```python
from build123d import *

# Parameters (mm, degrees)
SKETCH_1_W          = 49.5
SKETCH_1_H          = 24.5
EXTRUDE_1_DEPTH     = 22.5
SKETCH_2_R          = 2.5
CUT_EXTRUDE_1_DEPTH = 3
SKETCH_3_W          = 15.2
SKETCH_3_H          = 2.5
CUT_EXTRUDE_2_DEPTH = 8
CUT_EXTRUDE_3_DEPTH = 50
CUT_EXTRUDE_START   = 22.5
SKETCH_5_R          = 1.45
CUT_EXTRUDE_4_DEPTH = 10
FILLET_1_R          = 2.5


with BuildPart() as part:
    # Эскиз1 → Бобышка-Вытянуть1 (new body)
    with BuildSketch(Plane(origin=(0, 0, 0), x_dir=(0, 0, -1), z_dir=(1, 0, 0))):
        Rectangle(SKETCH_1_W, SKETCH_1_H)
    extrude(amount=EXTRUDE_1_DEPTH)

    # Эскиз2 → Вырез-Вытянуть1 (cut)
    with BuildSketch(Plane.ZY):
        with Locations((-20, -7.25)):
            Circle(SKETCH_2_R)
        with Locations((20, -7.25)):
            Circle(SKETCH_2_R)
    extrude(amount=-CUT_EXTRUDE_1_DEPTH, mode=Mode.SUBTRACT)

    # Эскиз3 → Вырез-Вытянуть2 (cut)
    with BuildSketch(Plane.ZY):
        with Locations((0, 8.75)):
            Rectangle(SKETCH_3_W, SKETCH_3_H)
    extrude(amount=-CUT_EXTRUDE_2_DEPTH, mode=Mode.SUBTRACT)

    # Эскиз4 → Вырез-Вытянуть3 (cut)
    with BuildSketch(Plane(origin=(0, 0, -24.75), x_dir=(-1, 0, 0), z_dir=(0, 0, -1))):
        with BuildLine():
            Line((-22.5, 12.25), (-22.5, -12.25))
            ThreePointArc((-22.5, -12.25), (-20.800548495, 0), (-22.5, 12.25))
        make_face()
    extrude(amount=-CUT_EXTRUDE_3_DEPTH, mode=Mode.SUBTRACT)

    # Эскиз5 → Вырез-Вытянуть4 (cut)
    with BuildSketch(Plane(origin=(0, 0, 0), x_dir=(0, 0, -1), z_dir=(1, 0, 0)).offset(CUT_EXTRUDE_START)):
        with Locations((-20, 0)):
            Circle(SKETCH_5_R)
        with Locations((20, 0)):
            Circle(SKETCH_5_R)
    extrude(amount=-CUT_EXTRUDE_4_DEPTH, mode=Mode.SUBTRACT)

    # Скругление1
    fillet_1_edges = [part.edges().sort_by_distance(p)[0] for p in [
        (11.25, 12.25, -24.75),
        (11.25, -12.25, -24.75),
        (11.25, -12.25, 24.75),
        (11.25, 12.25, 24.75),
    ]]
    fillet(fillet_1_edges, radius=FILLET_1_R)


solid = part.part
```
CAD build for the part. Positions are in the model's coordinates, mm. A direction names the side the tool comes from. Coordinates: 2 decimals unless noted, no trailing zeros. Write each loop counter-clockwise with the first axis right and the second up, starting at its lowest first coordinate (ties: lowest second). Pieces come first, ordered by that corner, then holes.
(1) Cut at D-D, the plane z = 20. List the corners of the cut face in (x, y).
(2) Cut at B-B, the plane z = -1. List the corners of the cut face in (x, y).
(3) Flat gauge pins, fed straight in: pin 1 (2.5 mm diameter, centred on y = 0, z = 19.5, fed in from +X); pin 2 (0.8 mm diameter, centred on y = 9.5, z = -2.5, fed in from -X); pin 3 (1.7 mm diameter, centred on y = 0, z = 20, fed in from -X); pin 4 (4.5 mm diameter, centred on y = -7.25, z = -20, fed in from -X). Where does each tip first touch, or does it go through?
(4) Drill centre lines: probe 1 along Y at (x, z) = (19, -20); probe 2 along Y at (x, z) = (1.25, 20); probe 3 along X at (y, z) = (-8.5, -5). Where is each one in solid material? Low to high.
(5) 3-axis set-ups, long thin cutter, end or side, ignore diameter. For faces 1 (the face through (4, 9, -7.6)), 2 (the face through (16.72, 0.44, 18.62)), 3 (the face through (20.8, -0.2, -0.3)): which of +Z, -Z, +X, -X, +Y, -Y reach the whole face in a straight line?
(6) Cut at C-C, the plane y = 0. List the corners of the cut face in (x, z), and give its area (3 significant figures).
(7) Cut at A-A, the plane x = 13.5. List the corners of the cut face in (y, z), and give its area (3 significant figures).
(8) Two-plate mould, pull along Y, no slides. Class faces 4 (the face through (11.408, -11.498, 24.037)), 5 (the face through (11.408, 11.498, 24.037)), 6 (the face through (1.479, -7.14, 17.502)): +Y half, -Y half, draft (parallel to the pull), parting line (faces both ways), or undercut.
Geometry says:
1. outline: (0, -12.25) - (22.5, -12.25) arc R45 cw to (20.82, -1.45) - (12.5, -1.45) - (12.5, 1.45) - (20.82, 1.45) arc R45 cw to (22.5, 12.25) - (0, 12.25) - (0, -4.75) - (3, -4.75) - (3, -9.75) - (0, -9.75) - close
2. outline: (0, -12.25) - (22.5, -12.25) arc R45 cw to (22.5, 12.25) - (0, 12.25) - (0, 10) - (8, 10) - (8, 7.5) - (0, 7.5) - close
3. pin 1: stops at x = 20.82
3. pin 2: stops at x = 8
3. pin 3: stops at x = 0
3. pin 4: stops at x = 3
4. probe 1: y = -12.25 to -1.45, 1.45 to 12.25
4. probe 2: y = -12.25 to -9.75, -4.75 to 12.25
4. probe 3: x = 0 to 21.61
5. face 1: -X
5. face 2: +X
5. face 3: +Z, -Z, +X
6. outline: (0, -24.75) - (20.8, -24.75) - (20.8, -21.45) - (12.5, -21.45) - (12.5, -18.55) - (20.8, -18.55) - (20.8, 18.55) - (12.5, 18.55) - (12.5, 21.45) - (20.8, 21.45) - (20.8, 24.75) - (0, 24.75) - close
6. area: 981 mm2
7. outline: (-12.25, -22.25) arc R2.5 ccw to (-9.75, -24.75) - (9.75, -24.75) arc R2.5 ccw to (12.25, -22.25) - (12.25, 22.25) arc R2.5 ccw to (9.75, 24.75) - (-9.75, 24.75) arc R2.5 ccw to (-12.25, 22.25) - close; hole circle Ø2.9 at (0, -20); hole circle Ø2.9 at (0, 20)
7. area: 1,190 mm2
8. face 4: -Y half
8. face 5: +Y half
8. face 6: undercut
